Source: CAD feature listing. Evaluate the final solid. Frame: model axes, mm. A direction names the side the tool comes from. Round coordinates to 2 decimals unless told otherwise and drop trailing zeros. Loops run counter-clockwise (first coordinate to the right, second up) from the corner with the lowest first, then second, coordinate; pieces in that order, holes last. Notation, with made-up numbers: (68, 20) - (93, 20) arc R19 cw to (93, 52) - close; hole circle Ø6 at (81.25, 87). An arc over 180 degrees is marked (long way). One line per question, with ' | ' between items. Start each with the question number.
1. Pin query (flat end, axial travel): pin 1 (10 mm diameter, centred on x = -7, y = -1.5, fed in from +Z); pin 2 (0.6 mm diameter, centred on x = 9.5, z = 71, fed in from +Y); pin 3 (2 mm diameter, centred on y = 0.5, z = 108, fed in from +X); pin 4 (1.2 mm diameter, centred on x = 1, z = 65.5, fed in from +Y). Return the tip coordinate at first contact, or that it passes through.
2. Ray query, line 1 (X direction, y = -5.5, z = 83); line 2 (X direction, y = 3.75, z = 51.5); line 3 (X direction, y = -9, z = 62). Return the intervals inside material, ascending.
3. Mould query, pull axis Y, two halves, no side actions, for faces 1 (the flat face through (6, -4, 118)), 2 (the cylindrical face through (-0.54, 2.44, 118.32)), 3 (the flat face through (2, -2, 240)), 4 (the flat face through (0, -4, 118)). Classes: pulls with the +Y half, pulls with the -Y half, needs draft (parallel to the pull), parting line crosses it, or undercut.
4. Access query for faces 5 (the flat face through (0, 4, 118)), 6 (the flat face through (10, -6, 118)), 7 (the flat face through (2, -2, 0)), 8 (the flat face through (-4, 0, 118)), 9 (the flat face through (4, 0, 118)). Directions: +Z, -Z, +X, -X, +Y, -Y. A direction counts if a zero-diameter tool reaches every point of the face in a straight line with its end or side. Return the directions, or none.
5. Cut plane A-A (x = 0). Return loops of the section in (y, z), then the cut area to 3 significant figures.
```python
from build123d import *

# Parameters (mm, degrees)
F1_DEPTH = 240
F2_R     = 1
F3_R     = 2.5
F4_DEPTH = 240


with BuildPart() as f1:
    # F0 (on Top) → F1 (new body)
    with BuildSketch(Plane.XY):
        Polygon((0, 4), (-2, 4), (-6, 8), (-3.5, 8.0038368255), (-3.5, 8.7538368255), (-2.5, 8.7538368255), (-2.5, 10.0038368255), (-10, 10), (-10, 2.4999990186), (-8.75, 2.4999990186), (-8.75, 3.4999990186), (-8, 3.4999990186), (-8, 5.9999990186), (-4, 2), (-4, 0), (-4, -2), (-8, -5.9999990186), (-8, -3.4999990186), (-8.75, -3.4999990186), (-8.75, -2.4999990186), (-10, -2.4999990186), (-10, -10), (-2.5, -10.0038368255), (-2.5, -8.7538368255), (-3.5, -8.7538368255), (-3.5, -8.0038368255), (-6, -8), (-2, -4), (0, -4), (2, -4), (6, -8), (3.5, -8.0038368255), (3.5, -8.7538368255), (2.5, -8.7538368255), (2.5, -10.0038368255), (10, -10), (10, -2.4999990186), (8.75, -2.4999990186), (8.75, -3.4999990186), (8, -3.4999990186), (8, -5.9999990186), (4, -2), (4, 0), (4, 2), (8, 5.9999990186), (8, 3.4999990186), (8.75, 3.4999990186), (8.75, 2.4999990186), (10, 2.4999990186), (10, 10), (2.5, 10.0038368255), (2.5, 8.7538368255), (3.5, 8.7538368255), (3.5, 8.0038368255), (6, 8), (2, 4), align=None)
    extrude(amount=F1_DEPTH)

    # F2
    f2_edges = [f1.edges().sort_by_distance(p)[0] for p in [
        (-10, -10, 120),
        (10, -10, 120),
        (-10, 10, 120),
        (10, 10, 120),
    ]]
    fillet(f2_edges, radius=F2_R)

    # F3 (on face) → F4 (cut, through all)
    with BuildSketch(Plane(origin=(0, 0, 0), x_dir=(1, 0, 0), z_dir=(0, 0, -1))):
        Circle(F3_R)
    extrude(amount=-F4_DEPTH, mode=Mode.SUBTRACT)


solid = f1.part
```
Answers follow:
1) pin 1: stops at z = 240 | pin 2: stops at y = 9.98 | pin 3: stops at x = 4 | pin 4: stops at y = 4
2) line 1: x = -10 to -8, -7.5 to -3.5, 3.5 to 7.5, 8 to 10 | line 2: x = -10 to -8, -5.75 to 5.75, 8 to 10 | line 3: x = -10 to -2.5, 2.5 to 10
3) face 1: undercut | face 2: undercut | face 3: needs draft | face 4: pulls with the -Y half
4) face 5: +Z, -Z, +Y | face 6: +Z, -Z, +X, +Y, -Y | face 7: -Z, +X, -X, +Y, -Y | face 8: +Z, -Z, -X | face 9: +Z, -Z, +X
5) outline: (-4, 0) - (-2.5, 0) - (-2.5, 240) - (-4, 240) - close; (2.5, 0) - (4, 0) - (4, 240) - (2.5, 240) - close | area: 720 mm2
